The model under review builds one solid part; all positions refer to its coordinate system, in mm. Coordinates: 2 decimals unless noted, no trailing zeros. Write each loop counter-clockwise with the first axis right and the second up, starting at its lowest first coordinate (ties: lowest second). Pieces come first, ordered by that corner, then holes.
1) For line 1 (Y direction, x = 11.5, z = -6.5); line 2 (X direction, y = 19.75, z = -22); line 3 (Y direction, x = 4.5, z = -14.25), list the stretches that pass through material, from the lowest coordinate up.
2) Add section A-A, the plane z = -23. State the section outline as (x, y) points.
3) Add section B-B, the plane y = 24. State the section outline as (x, z) points, then the cut area to 3 significant figures.
4) For P1, Ø4, axis at y = 22.5, z = -6.5, coming from the -X side, flat-tipped, find the tip position at first contact; note if it passes through.
5) Add section C-C, the plane x = 7. State the section outline as (y, z) points.
from build123d import *

# Parameters (mm, degrees)
F0_W     = 20
F0_H     = 14
F1_DEPTH = 25


with BuildPart() as f1:
    # F0 (on Top) → F1 (new body)
    with BuildSketch(Plane.XY):
        with Locations((6.421969, 12.208542)):
            Rectangle(F0_W, F0_H)
        Polygon((6.421969, 29.208542), (-3.578031, 19.208542), (16.421969, 19.208542), align=None)
    extrude(amount=-F1_DEPTH)


solid = f1.part
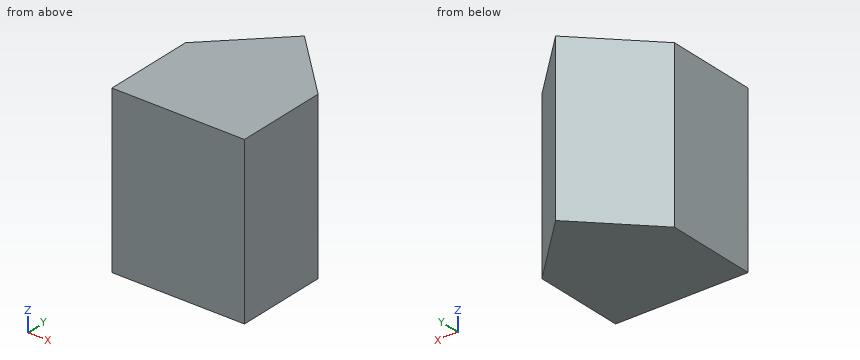
Geometry results:
1. line 1: y = 5.21 to 24.13
1. line 2: x = -3.04 to 15.88
1. line 3: y = 5.21 to 27.29
2. outline: (-3.58, 5.21) - (16.42, 5.21) - (16.42, 19.21) - (6.42, 29.21) - (-3.58, 19.21) - close
3. outline: (1.21, -25) - (11.63, -25) - (11.63, 0) - (1.21, 0) - close
3. area: 260 mm2
4. P1: stops at x = -2.29
5. outline: (5.21, -25) - (28.63, -25) - (28.63, 0) - (5.21, 0) - close
